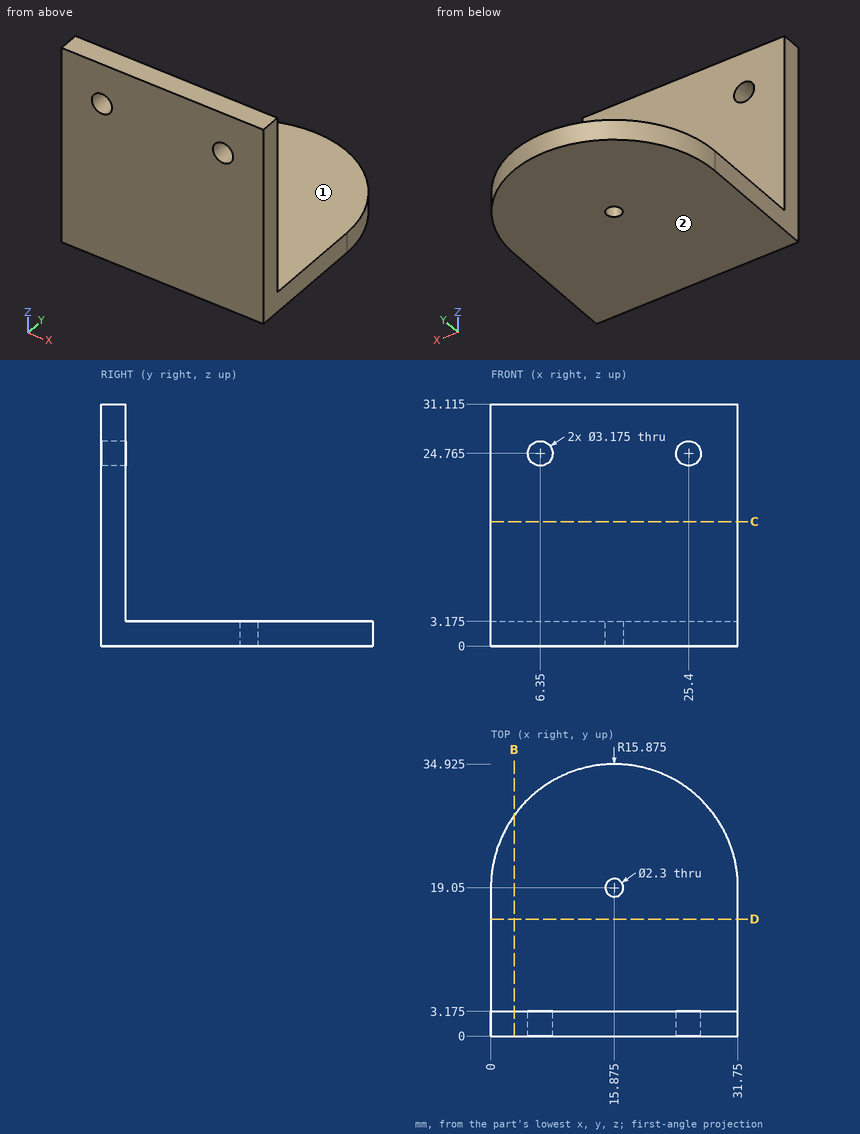
Print and shaded views of the part. All mm, measured from the part's lowest x, y and z. A direction names the side the tool comes from. Coordinates: 2 decimals unless noted, no trailing zeros. Loops run counter-clockwise (first coordinate to the right, second up) from the corner with the lowest first, then second, coordinate; pieces in that order, holes last. Notation, with made-up numbers: (54.25, 20) - (75.25, 20) arc R31 ccw to (75.25, 47) - close; hole circle Ø4 at (68, 62.25). An arc over 180 degrees is marked (long way). Write item = value, one per line. Start each with the question number.
Item 1: Cut at B-B, the plane x = 3. Give the cut face in (y, z) (3 decimals).
Item 2: 3-axis set-ups, long thin cutter, end or side, ignore diameter. For the marked faces 1 and 2: which of +Z, -Z, +X, -X, +Y, -Y reach the whole face in a straight line?
Item 3: Wall check: L1, parallel to Z at x = 25.4, y = 2.2 (1 decimal); L2, parallel to Z at x = 22.5, y = 12 (3 decimals). Give the ranges that are in metal, low to high. Write a range as from..to.
Item 4: Flat gauge pins, fed straight in: pin 1 Ø9.5 at (x, y) = (9, 17.5) entering from +Z (3 decimals); pin 2 Ø14 at (x, z) = (11.5, 11.5) entering from +Y (3 decimals). Where does each tip first touch, or does it go through?
Item 5: Cut at C-C, the plane z = 16. Give the cut face in (x, y) (3 decimals).
The answers:
q1.outline = (0, 0) - (28.337, 0) - (28.337, 3.175) - (3.175, 3.175) - (3.175, 31.115) - (0, 31.115) - close
q2.face_1 = +Z, +X, -X, +Y
q2.face_2 = -Z, +X, -X, +Y, -Y
q3.L1 = 0..23.2, 26.4..31.1
q3.L2 = 0..3.175
q4.pin_1 = 3.175
q4.pin_2 = 3.175
q5.outline = (0, 0) - (31.75, 0) - (31.75, 3.175) - (0, 3.175) - close
